Can you work these out from the model? Positions are in its coordinate system, mm. A direction names the side the tool comes from. Give positions to 0.01 mm unless a question says otherwise; leave off trailing zeros. Loops run counter-clockwise (first coordinate to the right, second up) from the corner with the lowest first, then second, coordinate; pieces in that order, holes last. Notation, with made-up numbers: M -21,65 L -1,65 A18 cw -1,72 Z; hole C 24,41 d2. An arc over 180 degrees is marked long. Answer as a JSON object with one key per item and string values.
```python
from build123d import *

# Parameters (mm, degrees)
SKETCH_2_R          = 12.5
EXTRUDE_3_DEPTH     = 375
SKETCH_5_R          = 3
CUT_EXTRUDE_2_DEPTH = 20
CUT_EXTRUDE_START   = -50
CUT_EXTRUDE_3_DEPTH = 50
EXTRUDE_START       = -20
SKETCH_11_R         = 12.5
EXTRUDE_5_DEPTH     = 20
CUT_EXTRUDE_START_2 = -20
SKETCH_12_R         = 3
CUT_EXTRUDE_4_DEPTH = 20
CHAMFER_1_SIZE      = 1
CHAMFER_2_SIZE      = 1


with BuildPart() as part:
    # 草图2 → 凸台-拉伸3 (new body)
    with BuildSketch(Plane(origin=(0, 0, 0), x_dir=(1, 0, 0), z_dir=(0, 1, 0))):
        with Locations(Location((0, 0, 0), (0, 0, 270))):
            Circle(SKETCH_2_R)
    extrude(amount=EXTRUDE_3_DEPTH)

    # 草图5 → 切除-拉伸2 (cut)
    with BuildSketch(Plane.XZ):
        with Locations(Location((0, 0, 0), (0, 0, 270))):
            Circle(SKETCH_5_R)
    extrude(amount=-CUT_EXTRUDE_2_DEPTH, mode=Mode.SUBTRACT)

    # 草图7 → 切除-拉伸3 (cut)
    with BuildSketch(Plane(origin=(0, 375, 0), x_dir=(1, 0, 0), z_dir=(0, 1, 0)).offset(CUT_EXTRUDE_START)):
        with BuildLine():
            Line((10, 7.5), (10, 0))
            Line((10, 0), (10, -7.5))
            ThreePointArc((10, -7.5), (11.858541226, -3.952847075), (12.5, 0))
            ThreePointArc((12.5, 0), (11.858541226, 3.952847075), (10, 7.5))
        make_face()
        with BuildLine():
            Line((-10, 0), (-10, 7.5))
            ThreePointArc((-10, 7.5), (-12.5, 0), (-10, -7.5))
            Line((-10, -7.5), (-10, 0))
        make_face()
    extrude(amount=CUT_EXTRUDE_3_DEPTH, mode=Mode.SUBTRACT)

    # 草图11 → 凸台-拉伸5 (add)
    with BuildSketch(Plane(origin=(0, 375, 0), x_dir=(1, 0, 0), z_dir=(0, 1, 0)).offset(EXTRUDE_START)):
        with Locations(Location((0, 0, 0), (0, 0, 270))):
            Circle(SKETCH_11_R)
    extrude(amount=EXTRUDE_5_DEPTH)

    # 草图12 → 切除-拉伸4 (cut)
    with BuildSketch(Plane(origin=(0, 375, 0), x_dir=(1, 0, 0), z_dir=(0, 1, 0)).offset(CUT_EXTRUDE_START_2)):
        with Locations(Location((0, 0, 0), (0, 0, 90))):
            Circle(SKETCH_12_R)
    extrude(amount=CUT_EXTRUDE_4_DEPTH, mode=Mode.SUBTRACT)

    # 倒角1
    chamfer_1_edges = [part.edges().sort_by_distance(p)[0] for p in [
        (0, 0, -12.5),
    ]]
    chamfer(chamfer_1_edges, length=CHAMFER_1_SIZE)

    # 倒角2
    chamfer_2_edges = [part.edges().sort_by_distance(p)[0] for p in [
        (0, 375, -12.5),
    ]]
    chamfer(chamfer_2_edges, length=CHAMFER_2_SIZE)


solid = part.part
```
1) Suppose I cut it at A-A, the plane y = 277.5. Write out the boundary of the cut face in (x, z).
Answer list:
{"outline": "C 0,0 d25"}
2) For faces 5 (the flat face through (-10, 340, 0)), 6 (the cylindrical face through (-0.9, 364.86, -2.86)), 7 (the flat face through (-2.4, 375, 2.4)), 8 (the flat face through (10, 340, 0)), which set-ups out of +Z, -Z, +X, -X, +Y, -Y let a thin tool reach every point of the face, with its end or its side?
Answer list:
{"face 5": "+Z, -Z, -X", "face 6": "+Y", "face 7": "+Z, -Z, +X, -X, +Y", "face 8": "+Z, -Z, +X"}
3) Please list where these lines run through material, in increasing order: line 1 along X through (y, z) = (368.5, 0); line 2 along Y through (x, z) = (0.75, 2); line 3 along X through (y, z) = (88.5, 7.5). Write a range as from..to.
Answer list:
{"line 1": "-12.5..-3, 3..12.5", "line 2": "20..355", "line 3": "-10..10"}
4) Will these pins go through, and if not, where does the flat tip stop? pin 1 Ø6 at (x, z) = (-8, 2) entering from -Y; pin 2 Ø5.5 at (x, z) = (0, 0) entering from +Y; pin 3 Ø3 at (x, y) = (6, 196.5) entering from +Z; pin 4 Ø5 at (y, z) = (46.5, 10) entering from -X.
Answer list:
{"pin 1": "y = 0", "pin 2": "y = 355", "pin 3": "z = 11.66", "pin 4": "x = -10"}
5) If we mould it in two halves opening along X, with no side actions, what happens to faces 1 (the cylindrical face through (0.55, 184.889, -12.488)), 2 (the cylindrical face through (0.9, 9.86, -2.86)), 3 (the flat face through (-2.4, 0, 2.4)), 4 (the flat face through (0, 20, 0))? For each: +X half, -X half, draft (parallel to the pull), parting line (faces both ways), or undercut.
Answer list:
{"face 1": "parting line", "face 2": "undercut", "face 3": "draft", "face 4": "undercut"}
